The listing builds one solid part. Answer for the finished solid, in the listing's coordinates (mm). Give positions to 0.01 mm unless a question says otherwise; leave off trailing zeros. Write each loop counter-clockwise with the first axis right and the second up, starting at its lowest first coordinate (ties: lowest second). Pieces come first, ordered by that corner, then holes. Notation, with made-up numbers: (7.25, -25.5) -> (21.25, -25.5) arc R18 cw to (21.25, -20.5) -> close; hole circle Ø11 at (-18.5, 55.25). An arc over 180 degrees is marked (long way). Write each question's results on one line, items separated by ' | '. Start each with the question number.
Autodesk Inventor part; units mm, degrees
ref_plane "YZ Plane" through (0, 0, 0) normal (1, 0, 0) x (0, 1, 0)
ref_plane "XZ Plane" through (0, 0, 0) normal (0, 1, 0) x (-1, 0, 0)
ref_plane "XY Plane" through (0, 0, 0) normal (0, 0, 1) x (1, 0, 0)
sketch "Sketch1" plane through (0, 0, 0) normal (0, 0, 1) x (1, 0, 0)
  circle A0 centre (-12.4986, 205.4088) radius 1.5
  circle A1 centre (-21.778, 213.3747) radius 1.5
  circle A2 centre (-28.3229, 203.0439) radius 1.5
  circle A3 centre (-19.0435, 195.0779) radius 1.5
  arc A4 (-18.8621, 189.3065) -> (-17.5296, 189.5057) centre (-17.9571, 187.8087) ccw
  arc A5 (-5.4909, 205.775) -> (-5.6901, 207.1075) centre (-3.9931, 206.68) ccw
  arc A6 (-35.3306, 202.6777) -> (-35.1315, 201.3452) centre (-36.8284, 201.7727) ccw
  arc A7 (-21.9594, 219.1462) -> (-23.2919, 218.947) centre (-22.8644, 220.644) ccw
  arc A8 (-19.2274, 216.8536) -> (-8.6812, 209.0499) centre (-10.7552, 217.2751) ccw
  arc A9 (-33.0381, 205.4097) -> (-25.2343, 215.9559) centre (-33.4595, 213.8819) ccw
  arc A10 (-21.5941, 191.5991) -> (-32.1403, 199.4028) centre (-30.0663, 191.1776) ccw
  arc A11 (-7.7835, 203.043) -> (-15.5873, 192.4968) centre (-7.362, 194.5708) ccw
  circle A12 centre (-3.9931, 206.68) radius 5.2556
  circle A13 centre (-22.8644, 220.644) radius 5.2531
  circle A14 centre (-36.8284, 201.7727) radius 5.2531
  circle A15 centre (-17.9571, 187.8087) radius 5.2531
  circle A16 centre (-3.9931, 206.68) radius 1.75
  circle A17 centre (-22.8644, 220.644) radius 1.75
  circle A18 centre (-36.8284, 201.7727) radius 1.75
  circle A19 centre (-17.9571, 187.8087) radius 1.75
  circle A20 centre (-20.4108, 204.2263) radius 4.75
  point P0 (0, 0)
  point P1 (-18.8621, 189.3065)
  point P2 (-17.5296, 189.5057)
  point P3 (-21.9594, 219.1462)
  point P4 (-23.2919, 218.947)
  point P5 (-5.4909, 205.775)
  point P6 (-5.6901, 207.1075)
  point P7 (-32.1403, 199.4028)
  point P8 (-21.5941, 191.5991)
  point P9 (-7.7868, 203.0428)
  point P10 (-8.6845, 209.0491)
  point P11 (-25.2343, 215.9559)
extrude "Extrusion1" add sketch "Sketch1" along normal blind 2
properties material "Steel"
1. Consider probe 1 along Y at (x, z) = (-27.5, 1.3); probe 2 along X at (y, z) = (211, 0.8); probe 3 along Y at (x, z) = (-15, 0.2). Determine where each line is inside the solid, lowest interval first. Write a range as [from, to].
2. Section B-B (y = 196) is taken. Write down the section's boundary in (x, z), then the cut area to 4 significant figures.
3. Section D-D (x = -34) is taken. Write down the section's boundary in (y, z).
4. Section C-C (x = -10.5) is taken. Write down the section's boundary in (y, z).
5. Section A-A (z = 1.7) is taken. Give the number of separate pieces and of enclosed holes in the cut face, then the cut area to 3 significant figures.
6. This flat-tipped pin is pushed along its axis until it touches: pin 1 Ø1 at (y, z) = (203.5, 0.5) entering from -X. Where does it stop, or does it pass through?
Results:
1) probe 1: y = [199.26, 201.79], [204.3, 207.85], [218.17, 223.12] | probe 2: x = [-25.48, -16.46], [-6.99, -1] | probe 3: y = [183.47, 192.15], [198.26, 209.93]
2) outline: (-23.09, 0) -> (-20.23, 0) -> (-20.23, 2) -> (-23.09, 2) -> close; (-17.86, 0) -> (-15.72, 0) -> (-15.72, 2) -> (-17.86, 2) -> close | area: 10.00 mm²
3) outline: (197.35, 0) -> (206.2, 0) -> (206.2, 2) -> (197.35, 2) -> close
4) outline: (202.45, 0) -> (208.8, 0) -> (208.8, 2) -> (202.45, 2) -> close
5) separate pieces: 1 | enclosed holes: 9 | area: 514 mm²
6) pin 1: stops at x = -41.94
